Could you check a few things on this model? Use its own coordinates, in mm. Give positions to 0.01 mm unless a question says otherwise; leave off trailing zeros. Loops run counter-clockwise (first coordinate to the right, second up) from the corner with the lowest first, then second, coordinate; pieces in that order, holes last. Notation, with made-up numbers: (41.25, -19.5) - (76.25, -19.5) arc R26 ccw to (76.25, 9.5) - close; hole circle Ø4 at (30, 52). An arc over 180 degrees is marked (long way). Write each question's results on one line, items separated by ' | '. Start each with the question number.
(1) Suppose I cut it at B-B (x = 79.5). Please give me the cut outline in (y, z), and give its area (3 significant figures).
(2) If we mould it in two halves opening along X, with no side actions, what happens to faces 1 (the face through (88.9, 63, -3)), 2 (the face through (41, 98.578, -3)), 3 (the face through (82.31, 39.69, -3.13))? For each: released by +X, released by -X, zero draft, split by the parting line, or undercut.
(3) I need wall thicknesses on line 1 (Y direction, x = 6, z = -4.25). Which ranges of the line are inside material? Lowest first, please.
(4) Suppose I cut it at A-A (y = 42). Please give me the cut outline in (x, z), and give its area (3 significant figures).
from build123d import *

# Parameters (mm, degrees)
SKETCH1_W           = 95.25
SKETCH1_H           = 70.374561309
BOSS_EXTRUDE1_DEPTH = 6.35
SKETCH2_R           = 3.175
CUT_EXTRUDE1_DEPTH  = 6.35


with BuildPart() as part:
    # Sketch1 → Boss-Extrude1 (new body)
    with BuildSketch(Plane.XY):
        with Locations((41.275, 63.390258975)):
            Rectangle(SKETCH1_W, SKETCH1_H)
    extrude(amount=-BOSS_EXTRUDE1_DEPTH)

    # Sketch2 → Cut-Extrude1 (cut)
    with BuildSketch(Plane.XY):
        with Locations((79.375, 40.90297832)):
            Circle(SKETCH2_R)
        with Locations((3.175, 40.90297832)):
            Circle(SKETCH2_R)
    extrude(amount=-CUT_EXTRUDE1_DEPTH, mode=Mode.SUBTRACT)


solid = part.part
Output values:
1) outline: (28.2, -6.35) - (37.73, -6.35) - (37.73, 0) - (28.2, 0) - close; (44.08, -6.35) - (98.58, -6.35) - (98.58, 0) - (44.08, 0) - close | area: 407 mm2
2) face 1: released by +X | face 2: zero draft | face 3: undercut
3) line 1: 28.2 to 39.45, 42.35 to 98.58
4) outline: (-6.35, -6.35) - (0.2, -6.35) - (0.2, 0) - (-6.35, 0) - close; (6.15, -6.35) - (76.4, -6.35) - (76.4, 0) - (6.15, 0) - close; (82.35, -6.35) - (88.9, -6.35) - (88.9, 0) - (82.35, 0) - close | area: 529 mm2
